```python
from build123d import *

# Parameters (mm, degrees)
SKETCH1_R           = 1.25
BOSS_EXTRUDE1_DEPTH = 15
SKETCH2_R           = 2.25
BOSS_EXTRUDE2_DEPTH = 3
CUT_EXTRUDE1_DEPTH  = 1.5


with BuildPart() as part:
    # Sketch1 → Boss-Extrude1 (new body)
    with BuildSketch(Plane.XY):
        Circle(SKETCH1_R)
    extrude(amount=-BOSS_EXTRUDE1_DEPTH)

    # Sketch2 → Boss-Extrude2 (add)
    with BuildSketch(Plane.XY):
        Circle(SKETCH2_R)
    extrude(amount=BOSS_EXTRUDE2_DEPTH)

    # Sketch3 → Cut-Revolve1 (revolve, cut)
    with BuildSketch(Plane(origin=(0, 0, 0), x_dir=(0, 0, -1), z_dir=(1, 0, 0)), mode=Mode.PRIVATE) as cut_revolve1_sk:
        with BuildLine():
            Line((-3, 2.15), (-3, 2.75))
            Line((-3, 2.75), (0, 2.75))
            Line((0, 2.75), (0, 2.15))
            Line((0, 2.15), (-0.5, 2.15))
            ThreePointArc((-0.5, 2.15), (-1.75, 2.25), (-3, 2.15))
        make_face()
    revolve(cut_revolve1_sk.sketch.rotate(Axis((0, 0, 3), (0, 0, 1)), 90), axis=Axis((0, 0, 3), (0, 0, 1)), mode=Mode.SUBTRACT)

    # Sketch4 → Cut-Extrude1 (cut)
    with BuildSketch(Plane.XY.offset(3)):
        Polygon((1.374815329, 0), (0.687407664, 1.190625), (-0.687407664, 1.190625), (-1.374815329, 0), (-0.687407664, -1.190625), (0.687407664, -1.190625), align=None)
    extrude(amount=-CUT_EXTRUDE1_DEPTH, mode=Mode.SUBTRACT)


solid = part.part
```
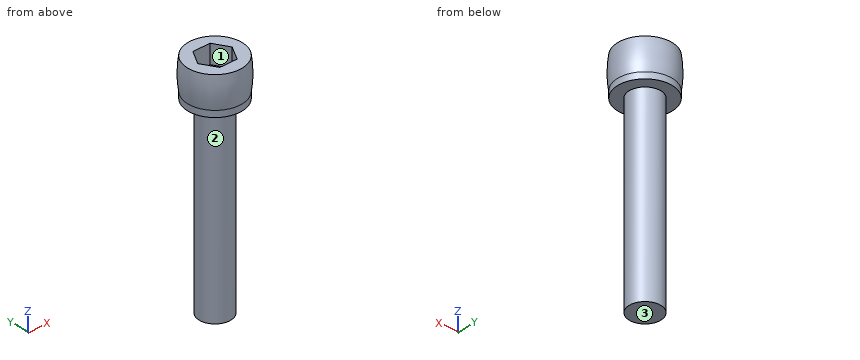
Could you check a few things on this model? Use its own coordinates, in mm. Face numbers are marked on the shaded views. Give positions to 0.01 mm unless a question says otherwise; leave off trailing zeros. Order: outer loops, then holes, each group sorted by start corner. A loop starts at its lowest first (then second) coordinate and runs counter-clockwise, first axis right, second up.
Q1. Suppose I cut it at A-A, the plane z = -6.25. Write out the boundary of the cut face in (x, y).
Q2. We'd pull the mould along X, two halves only. Please class the marked faces 1, 2 and 3: +X half, -X half, draft (parallel to the pull), parting line (faces both ways), or undercut.
Q3. If I drill on line 1 along Z through (x, y) = (-1.55, -0.2); line 2 along Z through (x, y) = (-0.4, -0.25); line 3 along Y through (x, z) = (-0.05, -4), over which ranges is the centre line in solid material (lowest first)?
Q4. I'm going to push flat-ended pins straight in: P1, Ø1.2, axis at x = -0.5, y = -0.5, coming from the +Z side; P2, Ø1, axis at x = 0.5, z = -13, coming from the +Y side. Where does each tip first touch, or does it pass through?
Solution:
1. outline: circle Ø2.5 at (0, 0)
2. face 1: undercut
2. face 2: parting line
2. face 3: draft
3. line 1: z = 0 to 3
3. line 2: z = -15 to 1.5
3. line 3: y = -1.25 to 1.25
4. P1: stops at z = 3
4. P2: stops at y = 1.25
